Geometry check sheet. Reference: the model listing, model coordinates, mm. Round coordinates to 2 decimals unless told otherwise and drop trailing zeros. Order: outer loops, then holes, each group sorted by start corner. A loop starts at its lowest first (then second) coordinate and runs counter-clockwise, first axis right, second up.
```python
from build123d import *

# Parameters (mm, degrees)
F1_DEPTH = 700
F2_R     = 15
F4_D     = 65
F4_DEPTH = 5
F4_TIP   = 19.5279701184


# Not quite as in the source:
# - a feature names something its author has since deleted; it is built from what else it names


with BuildPart() as f1:
    # F0 (on Right) → F1 (new body, symmetric)
    with BuildSketch(Plane.YZ):
        Polygon((-27.4648018735, 155.7606315443), (0, 0), (100, 0), (134.4682713554, 6.0776862183), (103.9881005213, 178.9393249289), align=None)
    extrude(amount=F1_DEPTH, both=True)

    # F2
    f2_edges = [f1.edges().sort_by_distance(p)[0] for p in [
        (0, 100, 0),
        (0, 134.468271, 6.077686),
        (0, 103.988101, 178.939325),
        (0, -27.464802, 155.760632),
        (0, 0, 0),
    ]]
    fillet(f2_edges, radius=F2_R)

    # F4
    with Locations(Plane(origin=(0, 0, 0), x_dir=(1, 0, 0), z_dir=(0, -0.984807753, -0.1736481777))):
        with Locations((-646, 108.1634903542), (-578, 108.1634903542), (-510, 108.1634903542), (-442, 108.1634903542), (-374, 108.1634903542), (-306, 108.1634903542), (-238, 108.1634903542), (-170, 108.1634903542), (-102, 108.1634903542), (-34, 108.1634903542), (34, 108.1634903542), (102, 108.1634903542), (170, 108.1634903542), (238, 108.1634903542), (306, 108.1634903542), (374, 108.1634903542), (442, 108.1634903542), (510, 108.1634903542), (578, 108.1634903542), (646, 108.1634903542)):
            Hole(F4_D / 2, depth=F4_DEPTH)
            with Locations((0, 0, -(F4_DEPTH + F4_TIP / 2))):  # 118° drill point
                Cone(0, F4_D / 2, F4_TIP, mode=Mode.SUBTRACT)


solid = f1.part
```
(1) Depth check by flat-ended pin: P1, Ø10, axis at x = -200.5, z = 109.5, coming from the +Y side; P2, Ø4, axis at x = 161, z = 30, coming from the -Y side; P3, Ø1, axis at x = -398.5, z = 86.5, coming from the +Y side. Enter the tip coordinate at first touch or a pass-through.
Returned:
P1: stops at y = 117.11
P2: stops at y = -5.64
P3: stops at y = 120.38
(2) Material ranges on line 1 (Z direction, x = -103, y = 93); line 2 (Z direction, x = 252, y = 19); line 3 (Y direction, x = 340, z = 53), recorded low to high.
Returned:
line 1: z = 0 to 176.52
line 2: z = 0 to 163.95
line 3: y = -9.35 to 126.19
(3) Sectioned sample at A-A, the plane y = 58. Record the cut outline in (x, z), and give its area (3 significant figures).
Returned:
outline: (-700, 0) - (700, 0) - (700, 170.83) - (-700, 170.83) - close
area: 239,000 mm2
(4) Draft check along Y on faces 1 (the flat face through (9.8, 119.405, 91.505)), 2 (the cylindrical face through (343.98, -14.12, 94.7)), 3 (the flat face through (-700, 52, 90)). Enter one of: released by +Y, released by -Y, zero draft, split by the parting line, or undercut.
Returned:
face 1: released by +Y
face 2: undercut
face 3: zero draft
(5) Sectioned sample at B-B, the plane z = 56. Record the cut outline in (x, y), and give its area (3 significant figures).
Returned:
outline: (-700, -9.87) - (700, -9.87) - (700, 125.67) - (-700, 125.67) - close
area: 190,000 mm2
